from build123d import *

# Parameters (mm, degrees)
BOSS_EXTRUDE1_DEPTH = 15.295
CUT_EXTRUDE1_DEPTH  = 206.919868261
FLOOR_START         = 3
FLOOR_2_DEPTH       = 3
BOSS_EXTRUDE4_START = 10.775
BOSS_EXTRUDE4_DEPTH = 10.775
BOSS_EXTRUDE5_REACH = 176.665
CUT_EXTRUDE3_REACH  = 209.578
SKETCH7_R           = 5.25
SKETCH14_OUTSIDE_W  = 59.009
SKETCH14_OUTSIDE_H  = 36.805
CUT_EXTRUDE4_DEPTH  = 33.295


with BuildPart() as part:
    # Sketch1 → Boss-Extrude1 (new body)
    with BuildSketch(Plane(origin=(0, 0, -12.295), x_dir=(-1, 0, 0), z_dir=(0, 0, -1))):
        with BuildLine():
            Line((-169.369133898, -111.490025098), (-130.678433581, -111.48937301))
            ThreePointArc((-130.678433581, -111.48937301), (-127.534095849, -100.145401406), (-130.522109497, -88.759255177))
            Line((-130.522109497, -88.759255177), (-169.350721063, -88.778648203))
            ThreePointArc((-169.350721063, -88.778648203), (-172.450070697, -100.131831373), (-169.369133898, -111.490025098))
        make_face()
    extrude(amount=-BOSS_EXTRUDE1_DEPTH)

    # Sketch2 → Cut-Extrude1 (cut, through all)
    with BuildSketch(Plane.XY.offset(3)):
        with BuildLine():
            Line((168.171133654, -90.778059306), (131.717568579, -90.759852501))
            ThreePointArc((131.717568579, -90.759852501), (129.534116109, -100.141151153), (131.855022492, -109.48939284))
            Line((131.855022492, -109.48939284), (168.187605365, -109.490005184))
            ThreePointArc((168.187605365, -109.490005184), (170.450070154, -100.132033398), (168.171133654, -90.778059306))
        make_face()
    extrude(amount=-CUT_EXTRUDE1_DEPTH, mode=Mode.SUBTRACT)

    # Sketch4 → floor 2 (add)
    with BuildSketch(Plane(origin=(0, 0, -12.295), x_dir=(-1, 0, 0), z_dir=(0, 0, -1)).offset(FLOOR_START)):
        with BuildLine():
            Line((-169.369133898, -111.490025098), (-130.678433581, -111.48937301))
            ThreePointArc((-130.678433581, -111.48937301), (-127.534095849, -100.145401406), (-130.522109497, -88.759255177))
            Line((-130.522109497, -88.759255177), (-169.350721063, -88.778648203))
            ThreePointArc((-169.350721063, -88.778648203), (-172.450070697, -100.131831373), (-169.369133898, -111.490025098))
        make_face()
    extrude(amount=-FLOOR_2_DEPTH)

    # Sketch6 → Boss-Extrude4 (add)
    with BuildSketch(Plane.XY.offset(-12.295).offset(BOSS_EXTRUDE4_START)):
        with BuildLine():
            Line((146.5, -90.767235615), (146.5, -108.989639664))
            Line((146.5, -108.989639664), (168.187605365, -109.490005184))
            ThreePointArc((168.187605365, -109.490005184), (170.450070154, -100.132033398), (168.171133654, -90.778059306))
            Line((168.171133654, -90.778059306), (146.5, -90.767235615))
        make_face()
    extrude(amount=-BOSS_EXTRUDE4_DEPTH)

    # Boss-Extrude5: up to this face of the body (flat: up to its plane)
    boss_extrude5_end = Plane(part.part.faces().sort_by_distance((150.023783739, -111.489699054, -6.1475))[0])
    # Sketch11 → Boss-Extrude5 (add, up to the picked face)
    with BuildSketch(Plane(origin=(-0.044298414, -88.694043528, 0), x_dir=(0.9999998752738909, -0.0004994519023308322, 0), z_dir=(0.0004994519023308322, 0.9999998752738909, 0)), mode=Mode.PRIVATE) as boss_extrude5_sk1:
        Polygon((150.03815576, 15.295), (166.500079456, 30.295), (172.500079456, 30.295), (172.500079456, 15.295), align=None)
    boss_extrude5_tool1 = split(extrude(boss_extrude5_sk1.sketch, amount=-BOSS_EXTRUDE5_REACH, mode=Mode.PRIVATE), bisect_by=boss_extrude5_end, keep=Keep.BOTH, mode=Mode.PRIVATE)
    boss_extrude5 = boss_extrude5_tool1.solids().sort_by(Axis((164.546837, -88.776249, -21.34904), (-0.0004994519023308322, -0.9999998752738909, 0)))[0]
    add(boss_extrude5)

    # Cut-Extrude3: up to this face of the body (flat: up to its plane)
    cut_extrude3_end = Plane(part.part.faces().sort_by_distance((146.5, -99.87843764, -6.9075))[0])
    # Sketch7 → Cut-Extrude3 (cut, up to the picked face)
    with BuildSketch(Plane(origin=(0, 0, 0), x_dir=(0, 0, -1), z_dir=(1, 0, 0)), mode=Mode.PRIVATE) as cut_extrude3_sk1:
        with Locations(Location((7.995, -100, 0), (0, 0, 180))):
            Circle(SKETCH7_R)
    cut_extrude3_tool1 = split(extrude(cut_extrude3_sk1.sketch, amount=CUT_EXTRUDE3_REACH, mode=Mode.PRIVATE), bisect_by=cut_extrude3_end, keep=Keep.BOTH, mode=Mode.PRIVATE)
    add(cut_extrude3_tool1.solids().sort_by(Axis((0, -100, -7.995), (1, 0, 0)))[0], mode=Mode.SUBTRACT)

    # Mirror1: Boss-Extrude5 across plane
    add(boss_extrude5.mirror(Plane(origin=(149.98984246, -0.002527909, 0), x_dir=(0, 0, 1), z_dir=(-0.9999999998579736, 1.6853871084051315e-05, 0))))

    # Sketch14 outside → Cut-Extrude4 (cut)
    with BuildSketch(Plane.XY.offset(3)):
        with Locations((149.9885, -100.1245)):
            Rectangle(SKETCH14_OUTSIDE_W, SKETCH14_OUTSIDE_H)
        with BuildLine():
            Line((169.350721063, -88.778648203), (130.522109497, -88.759255177))
            ThreePointArc((130.522109497, -88.759255177), (127.534095849, -100.145401406), (130.678433581, -111.48937301))
            Line((130.678433581, -111.48937301), (169.369133898, -111.490025098))
            ThreePointArc((169.369133898, -111.490025098), (172.450070697, -100.131831373), (169.350721063, -88.778648203))
        make_face(mode=Mode.SUBTRACT)
    extrude(amount=-CUT_EXTRUDE4_DEPTH, mode=Mode.SUBTRACT)


with BuildPart() as part_1:
    # Body-Move/Copy1: moved
    add(part.part.moved(Location((-149.988154595, 100.149527643, 15.295))))


solid = part_1.part
CAD build for the part. Positions are in the model's coordinates, mm. A direction names the side the tool comes from. Round coordinates to 2 decimals unless told otherwise and drop trailing zeros. Write each loop counter-clockwise with the first axis right and the second up, starting at its lowest first coordinate (ties: lowest second). Pieces come first, ordered by that corner, then holes. Notation, with made-up numbers: M 76.25,50.5 L 95.25,50.5 A6 ccw 95.25,59.5 Z; hole C 64.25,-24 d9. An arc over 180 degrees is marked long. Use a Markdown table: item, result. Add a question column.
1. Slice it at C-C on x = 3. Give the cut face in (y, z) (3 decimals), then the cut area to 3 significant figures.
2. 3-axis set-ups, long thin cutter, end or side, ignore diameter. For faces 5 (the face through (2, 10, 18.295)), 6 (the face through (-15.12, 0.07, 2.05)), 7 (the face through (20.46, -0.12, 16.07)): which of +Z, -Z, +X, -X, +Y, -Y reach the whole face in a straight line?
3. Pull direction X, two halves, no side cores. Call faces 1 (the face through (-22.455, 0.171, 1.881)), 2 (the face through (-9, -6, 3)), 3 (the face through (-19, 0, -15)), 4 (the face through (8, 0, 13.775)): released by +X, released by -X, zero draft, split by the parting line, or undercut.
4. Slice it at A-A on y = 4.75. Give the cut face in (x, z) (3 decimals).
5. Slice it at D-D on y = 7.25. Give the cut face in (x, z) (3 decimals).
6. Drill centre lines: probe 1 along Y at (x, z) = (-13, 7); probe 2 along X at (y, z) = (-6, -11); probe 3 along X at (y, z) = (7.5, -12.5). Where is each one in solid material? Low to high.
7. Slice it at B-B on z = 7.3. Give the cut face in (x, y), then the cut area to 3 significant figures.
8. Flat gauge pins, fed straight in: P1, Ø4, axis at x = -3, y = -0.5, coming from the -Z side; P2, Ø2, axis at y = 2, z = 7, coming from the +X side; P3, Ø1.5, axis at y = -8, z = 14.5, coming from the +X side. Where does each tip first touch, or does it go through?
Reply:
| question | item | result |
|---|---|---|
| 1 | outline | M -11.34,-2.739 L 11.379,-2.728 L 11.379,18.295 L 9.379,18.295 L 9.379,13.775 L -8.99,13.775 L -8.99,3 L -9.34,3 L -9.34,18.295 L -11.34,18.295 Z |
| 1 | area | 389 mm^2 |
| 2 | face 5 | +Z, +X, -X, +Y, -Y |
| 2 | face 6 | -X |
| 2 | face 7 | +Z |
| 3 | face 1 | released by -X |
| 3 | face 2 | undercut |
| 3 | face 3 | zero draft |
| 3 | face 4 | undercut |
| 4 | outline | M -21.983,-15 L -16.464,-15 L -0.002,0 L 0.002,0 L 16.464,-15 L 21.953,-15 L 21.953,18.295 L 19.901,18.295 L 19.901,13.775 L -3.488,13.775 L -3.488,3 L -19.937,3 L -19.937,4.771 L -21.983,4.771 Z; M -21.983,9.829 L -19.937,9.829 L -19.937,18.295 L -21.983,18.295 Z |
| 5 | outline | M -21.313,-15 L -16.465,-15 L -0.003,0 L 0.004,0 L 16.466,-15 L 21.257,-15 L 21.257,18.295 L 19.131,18.295 L 19.131,13.775 L -3.488,13.775 L -3.488,3 L -19.196,3 L -19.196,18.295 L -21.313,18.295 Z |
| 6 | probe 1 | y = -11.34 to -9.34, 9.39 to 11.39 |
| 6 | probe 2 | x = -21.6 to -12.07, 12.07 to 21.64 |
| 6 | probe 3 | x = -21.23 to -13.72, 13.72 to 21.17 |
| 7 | outline | M -21.84,5.4 L -19.78,5.4 A20.6 cw -18.27,9.39 L -3.49,9.38 L -3.49,-8.84 L 18.2,-9.34 L -18.13,-9.34 A20.6 cw -19.77,-5.1 L -21.83,-5.1 A22.6 ccw -19.31,-11.34 L 19.38,-11.34 A22.41 ccw 19.36,11.37 L -19.47,11.39 A22.6 ccw Z |
| 7 | area | 645 mm^2 |
| 8 | P1 | stops at z = -4.56 |
| 8 | P2 | stops at x = 22.44 |
| 8 | P3 | stops at x = 21.26 |
